```python
from build123d import *

# Parameters (mm, degrees)
SKETCH_R            = 2.25
BOSS_EXTRUDE3_DEPTH = 40
SKETCH1_W           = 249.949747468
SKETCH1_H           = 30
CUT_EXTRUDE1_DEPTH  = 25


with BuildPart() as part:
    # Sketch → Boss-Extrude3 (new body)
    with BuildSketch(Plane(origin=(0, 0, 0), x_dir=(1, 0, 0), z_dir=(0, 1, 0))):
        with BuildLine():
            Line((0, 191.780935723), (250, 191.780935723))
            Line((250, 191.780935723), (250, 133.455634672))
            ThreePointArc((250, 133.455634672), (247.75, 131.205634672), (250, 128.955634672))
            Line((250, 128.955634672), (250, -268.294365328))
            Line((250, -268.294365328), (125, -268.294365328))
            Line((125, -268.294365328), (125, -343.294365328))
            Line((125, -343.294365328), (250, -343.294365328))
            Line((250, -343.294365328), (250, -740.544365328))
            ThreePointArc((250, -740.544365328), (247.75, -742.794365328), (250, -745.044365328))
            Line((250, -745.044365328), (250, -803.36966638))
            Line((250, -803.36966638), (0, -803.36966638))
            Line((0, -803.36966638), (0, -750))
            Line((0, -750), (120, -750))
            Line((120, -750), (120, -610))
            Line((120, -610), (0, -610))
            Line((0, -610), (0, -1.588730657))
            Line((0, -1.588730657), (120, -1.588730657))
            Line((120, -1.588730657), (120, 138.411269343))
            Line((120, 138.411269343), (0, 138.411269343))
            Line((0, 138.411269343), (0, 191.780935723))
        make_face()
        with Locations((125, 131.205634672)):
            Circle(SKETCH_R, mode=Mode.SUBTRACT)
        with Locations((150, 131.205634672)):
            Circle(SKETCH_R, mode=Mode.SUBTRACT)
        with Locations((175, 131.205634672)):
            Circle(SKETCH_R, mode=Mode.SUBTRACT)
        with Locations((200, 131.205634672)):
            Circle(SKETCH_R, mode=Mode.SUBTRACT)
        with Locations((225, 131.205634672)):
            Circle(SKETCH_R, mode=Mode.SUBTRACT)
        with Locations((225, -742.794365328)):
            Circle(SKETCH_R, mode=Mode.SUBTRACT)
        with Locations((200, -742.794365328)):
            Circle(SKETCH_R, mode=Mode.SUBTRACT)
        with Locations((175, -742.794365328)):
            Circle(SKETCH_R, mode=Mode.SUBTRACT)
        with Locations((150, -742.794365328)):
            Circle(SKETCH_R, mode=Mode.SUBTRACT)
        with Locations((125, -742.794365328)):
            Circle(SKETCH_R, mode=Mode.SUBTRACT)
        with BuildLine():
            ThreePointArc((50.51221471, -290.298610608), (50, -286.225703188), (49.48778529, -290.298610608))
            ThreePointArc((49.48778529, -290.298610608), (34.497008873, -305.989414978), (49.877802923, -321.29810185))
            ThreePointArc((49.877802923, -321.29810185), (50, -325.294365328), (50.122197077, -321.29810185))
            ThreePointArc((50.122197077, -321.29810185), (65.502991127, -305.989414978), (50.51221471, -290.298610608))
        make_face(mode=Mode.SUBTRACT)
    extrude(amount=BOSS_EXTRUDE3_DEPTH)

    # Sketch1 → Cut-Extrude1 (cut)
    with BuildSketch(Plane(origin=(0, 40, 0), x_dir=(1, 0, 0), z_dir=(0, 1, 0))):
        with Locations((125.025126266, 130)):
            Rectangle(SKETCH1_W, SKETCH1_H)
        with Locations((125.025126266, -741.588730657)):
            Rectangle(SKETCH1_W, SKETCH1_H)
    extrude(amount=-CUT_EXTRUDE1_DEPTH, mode=Mode.SUBTRACT)


solid = part.part
```
Input: part model. Units: mm. Frame: model coordinates. A direction names the side the tool comes from. Give positions to 0.01 mm unless a question says otherwise; leave off trailing zeros. Order: outer loops, then holes, each group sorted by start corner. A loop starts at its lowest first (then second) coordinate and runs counter-clockwise, first axis right, second up.
1. Section C-C on z = -26. Return the cut outline in (x, y), and give its area (3 significant figures).
Derived:
outline: (120, 0) - (250, 0) - (250, 40) - (120, 40) - close
area: 5,200 mm2
2. Section A-A on y = 27.5. Return the cut outline in (x, z), and give its area (3 significant figures).
Derived:
outline: (0, -191.78) - (250, -191.78) - (250, -145) - (0.05, -145) - (0.05, -138.41) - (0, -138.41) - close; (0, 1.59) - (120, 1.59) - (120, -115) - (250, -115) - (250, 268.29) - (125, 268.29) - (125, 343.29) - (250, 343.29) - (250, 726.59) - (120, 726.59) - (120, 610) - (0, 610) - close; (0, 750) - (0.05, 750) - (0.05, 756.59) - (250, 756.59) - (250, 803.37) - (0, 803.37) - close; hole (49.49, 290.3) arc R2.07 ccw (long way) to (50.51, 290.3) arc R15.5 ccw to (50.12, 321.3) arc R2 ccw (long way) to (49.88, 321.3) arc R15.5 ccw to start
area: 196,000 mm2
3. Mould query, pull axis Z, two halves, no side actions, for faces 6 (the flat face through (123, 20, -191.781)), 7 (the flat face through (120, 20, -67)), 8 (the flat face through (99, 40, 300)). Classes: released by +Z, released by -Z, zero draft, split by the parting line, or undercut.
Derived:
face 6: released by -Z
face 7: undercut
face 8: zero draft
4. Material intervals for L1, parallel to Z at x = 98, y = 33.5; L2, parallel to Z at x = 116, y = 2; L3, parallel to Z at x = 202.5, y = 16, sorted ascending.
Derived:
L1: z = -191.78 to -145, 1.59 to 610, 756.59 to 803.37
L2: z = -191.78 to -138.41, 1.59 to 610, 750 to 803.37
L3: z = -191.78 to -145, -115 to 268.29, 343.29 to 726.59, 756.59 to 803.37
5. Reachability of faces 1 (the flat face through (151, 15, -134)), 2 (the flat face through (184, 28, -115)), 3 (the flat face through (188, 20, 268.294)), 4 (the flat face through (61, 20, 610)), 5 (the cylindrical face through (65.495, 19.72, 306.326)) from +Z, -Z, +X, -X, +Y, -Y: full face, straight path, thin tool, end or side. Return the list, or none.
Derived:
face 1: +X, +Y
face 2: +X, -X, +Y
face 3: +X, +Y, -Y
face 4: -X, +Y, -Y
face 5: +Y, -Y
6. Pin query (flat end, axial travel): pin 1 (8 mm diameter, centred on y = 31.5, z = -31, fed in from -X); pin 2 (6 mm diameter, centred on x = 200, z = -131.21, fed in from +Y); pin 3 (2 mm diameter, centred on y = 33.5, z = 753, fed in from +X). Return the tip coordinate at first contact, or that it passes through.
Derived:
pin 1: stops at x = 120
pin 2: stops at y = 15
pin 3: stops at x = 0.05
7. Section B-B on z = 303. Return the cut outline in (x, y), and give its area (3 significant figures).
Derived:
outline: (0, 0) - (34.75, 0) - (34.75, 40) - (0, 40) - close; (65.25, 0) - (125, 0) - (125, 40) - (65.25, 40) - close
area: 3,780 mm2
